Read the model definition and answer for the solid it produces. Units are mm, in the model's axes. A direction names the side the tool comes from. Coordinates: 2 decimals unless noted, no trailing zeros. Order: outer loops, then holes, each group sorted by start corner. A loop starts at its lowest first (then second) coordinate and runs counter-clockwise, first axis right, second up. Notation, with made-up numbers: M 7.25,-11.5 L 48.25,-11.5 A28 ccw 48.25,6.5 Z; hole C 64,59.5 d9. An arc over 180 degrees is marked long. Use a Markdown table: item, result. Add a question column.
1) Find the intervals of material crossed by probe 1 along X at (y, z) = (18, 19.5); probe 2 along X at (y, z) = (28.5, 19); probe 3 along Z at (x, y) = (78, 3), in increasing order. Write a range as [from, to].
2) Find section D-D on x = 20. Write down the section's boundary in (y, z), plus the area to 3 significant figures.
3) Find section B-B on x = 6. Write down the section's boundary in (y, z), plus the area to 3 significant figures.
4) For faces 4 (the face through (20.275, 28.225, 17.503)), 5 (the face through (100, 12, 15)), determine the directions among +Z, -Z, +X, -X, +Y, -Y from which every point of the face is accessible in a straight line to the end or side of a thin tool.
5) The mould has two halves that part along X. Classify faces 1 (the face through (65, 6, 30)), 2 (the face through (0, 28, 15)), 3 (the face through (50.275, 22.902, 17.503)): released by +X, released by -X, zero draft, split by the parting line, or undercut.
6) Find section A-A on y = 20. Write down the section's boundary in (x, z), plus the area to 3 significant figures.
7) Find section C-C on z = 14.5. Write down the section's boundary in (x, y).
8) Each of these flat-tipped pins is pushed along its axis until it touches: pin 1 Ø2 at (x, z) = (16, 7) entering from -Y; pin 2 Ø6 at (x, y) = (49.5, 6) entering from +Z; pin 3 Ø12 at (x, z) = (71.5, 9.5) entering from -Y. Where does it stop, or does it pass through?
from build123d import *

# Parameters (mm, degrees)
EXTRUDE1_DEPTH    = 30
EXTRUDE2_REACH    = 136.629
SKETCH2_R         = 12.5
LPATTERN1_START   = -0.809693491
LPATTERN1_DEPTH   = 55.809693491
LPATTERN1_START_2 = -9.809693491
LPATTERN1_2_DEPTH = 55.831993491
LPATTERN1_START_3 = -17.309693491
LPATTERN1_3_DEPTH = 7.5
LPATTERN1_START_4 = -8.309693491
LPATTERN1_4_DEPTH = 7.5
LPATTERN1_START_5 = 17
LPATTERN1_5_DEPTH = 13


with BuildPart() as part:
    # Sketch1 → Extrude1 (new body)
    with BuildSketch(Plane.XY):
        Polygon((0, 0), (100, -30), (100, 55), (0, 55), align=None)
    extrude(amount=EXTRUDE1_DEPTH)

    # Extrude2: up to this plane
    extrude2_end = Plane(origin=(2.873478856, 9.578262852, 30), z_dir=(0.2873478855663455, 0.9578262852211514, 0))
    # Sketch2 → Extrude2 (cut, up to the surface)
    with BuildSketch(Plane(origin=(0, 55, 0), x_dir=(1, 0, 0), z_dir=(0, 1, 0)), mode=Mode.PRIVATE) as extrude2_sk1:
        with Locations((20, -30)):
            Circle(SKETCH2_R)
    extrude2_tool1 = split(extrude(extrude2_sk1.sketch, amount=-EXTRUDE2_REACH, mode=Mode.PRIVATE), bisect_by=extrude2_end, keep=Keep.BOTH, mode=Mode.PRIVATE)
    add(extrude2_tool1.solids().sort_by_distance((20, 55, 30))[0], mode=Mode.SUBTRACT)

    # LPattern1: read off the stored shape, not the designer's step
    # LPattern1 outline → LPattern1 (cut)
    with BuildSketch(Plane(origin=(0, 0, 0), x_dir=(1, 0, 0), z_dir=(0, 1, 0)).offset(LPATTERN1_START)):
        with BuildLine():
            Line((37.5, -30), (62.5, -30))
            ThreePointArc((62.5, -30), (50, -17.5), (37.5, -30))
        make_face()
        with BuildLine():
            ThreePointArc((92.5, -30), (80, -17.5), (67.5, -30))
            Line((67.5, -30), (92.5, -30))
        make_face()
    extrude(amount=LPATTERN1_DEPTH, mode=Mode.SUBTRACT)

    # LPattern1 2 outline → LPattern1 2 (cut)
    with BuildSketch(Plane(origin=(0, 0, 0), x_dir=(1, 0, 0), z_dir=(0, 1, 0)).offset(LPATTERN1_START_2)):
        with BuildLine():
            ThreePointArc((92.5, -30), (80, -17.5), (67.5, -30))
            Line((67.5, -30), (92.5, -30))
        make_face()
    extrude(amount=LPATTERN1_2_DEPTH, mode=Mode.SUBTRACT)

    # LPattern1 3 outline → LPattern1 3 (cut)
    with BuildSketch(Plane(origin=(0, 0, 0), x_dir=(1, 0, 0), z_dir=(0, 1, 0)).offset(LPATTERN1_START_3)):
        with BuildLine():
            ThreePointArc((92.5, -30), (80, -17.5), (67.5, -30))
            Line((67.5, -30), (92.5, -30))
        make_face()
    extrude(amount=LPATTERN1_3_DEPTH, mode=Mode.SUBTRACT)

    # LPattern1 4 outline → LPattern1 4 (cut)
    with BuildSketch(Plane(origin=(0, 0, 0), x_dir=(1, 0, 0), z_dir=(0, 1, 0)).offset(LPATTERN1_START_4)):
        with BuildLine():
            Line((37.5, -30), (62.5, -30))
            ThreePointArc((62.5, -30), (50, -17.5), (37.5, -30))
        make_face()
    extrude(amount=LPATTERN1_4_DEPTH, mode=Mode.SUBTRACT)

    # LPattern1 5 outline → LPattern1 5 (add)
    with BuildSketch(Plane.XY.offset(LPATTERN1_START_5)):
        Polygon((92.5, 55), (92.5, -17.309693491), (67.5, -9.809693491), (67.5, 55), (62.5, 55), (62.5, -8.309693491), (37.5, -0.809693491), (37.5, 55), (32.5, 55), (32.5, 0.690306509), (7.5, 8.190306509), (7.5, 55), (0, 55), (0, 0), (100, -30), (100, 55), align=None)
    extrude(amount=LPATTERN1_5_DEPTH)


solid = part.part
Check result:
| question | item | result |
|---|---|---|
| 1 | probe 1 | x = [0, 13.22], [26.78, 43.22], [56.78, 73.22], [86.78, 100] |
| 1 | probe 2 | x = [0, 14.06], [25.94, 44.06], [55.94, 74.06], [85.94, 100] |
| 1 | probe 3 | z = [0, 17.66] |
| 2 | outline | M -6,0 L 55,0 L 55,17.5 L 4.44,17.5 L 4.44,30 L -6,30 Z |
| 2 | area | 1,200 mm2 |
| 3 | outline | M -1.8,0 L 55,0 L 55,30 L -1.8,30 Z |
| 3 | area | 1,700 mm2 |
| 4 | face 4 | +Z, +Y |
| 4 | face 5 | +Z, -Z, +X, +Y, -Y |
| 5 | face 1 | zero draft |
| 5 | face 2 | released by -X |
| 5 | face 3 | undercut |
| 6 | outline | M 0,0 L 100,0 L 100,30 L 92.5,30 A12.5 cw 67.5,30 L 62.5,30 A12.5 cw 37.5,30 L 32.5,30 A12.5 cw 7.5,30 L 0,30 Z |
| 6 | area | 2,260 mm2 |
| 7 | outline | M 0,0 L 100,-30 L 100,55 L 0,55 Z |
| 8 | pin 1 | stops at y = -5.1 |
| 8 | pin 2 | stops at z = 18 |
| 8 | pin 3 | stops at y = -23.25 |
